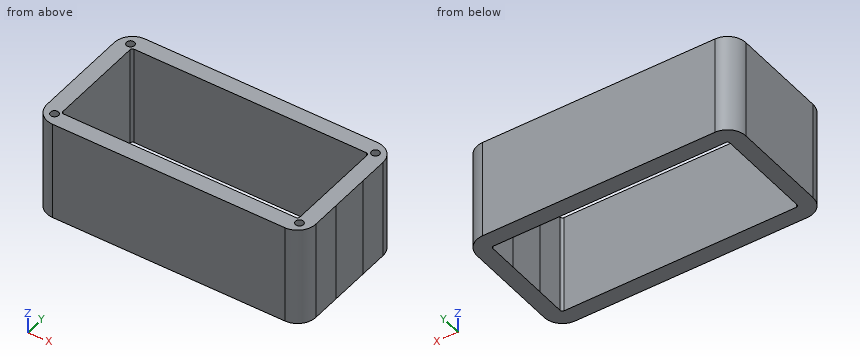
Autodesk Inventor part; units mm, degrees
ref_plane "YZ Plane" through (0, 0, 0) normal (1, 0, 0) x (0, 1, 0)
ref_plane "XZ Plane" through (0, 0, 0) normal (0, 1, 0) x (-1, 0, 0)
ref_plane "XY Plane" through (0, 0, 0) normal (0, 0, 1) x (1, 0, 0)
sketch "Sketch1" plane through (0, 0, 0) normal (0, 0, 1) x (1, 0, 0)
  line L0 (63.4168, -84.0015) -> (-66.0832, -83.9994)
  line L1 (63.4168, -84.0015) -> (81.9168, -84.0018)
  line L2 (-67.5831, -82.4994) -> (-67.5821, -20.9994)
  arc A0 (-67.5831, -82.4994) -> (-66.0832, -83.9994) centre (-66.0831, -82.4994) ccw
  arc A1 (-66.0821, -19.4994) -> (-67.5821, -20.9994) centre (-66.0821, -20.9994) ccw
  line L3 (-66.0821, -19.4994) -> (63.4179, -19.5015)
  line L4 (64.1679, -20.2516) -> (81.9179, -20.2518)
  line L5 (81.9179, -19.5018) -> (63.4179, -19.5015)
  arc A2 (83.4179, -21.0019) -> (81.9179, -19.5018) centre (81.9179, -21.0018) ccw
  line L6 (83.4176, -39.5019) -> (83.4179, -21.0019)
  line L7 (83.4176, -39.5019) -> (83.4172, -64.0019)
  line L8 (83.4169, -82.5019) -> (83.4172, -64.0019)
  arc A3 (81.9168, -84.0018) -> (83.4169, -82.5019) centre (81.9169, -82.5018) ccw
  line L9 (-77.7421, -20.9992) -> (-77.7431, -82.4992)
  arc A4 (-77.7431, -82.4992) -> (-66.0833, -94.1594) centre (-66.0831, -82.4994) ccw
  line L10 (-66.0833, -94.1594) -> (63.4167, -94.1615)
  line L11 (63.4167, -94.1615) -> (81.9167, -94.1618)
  arc A5 (81.9167, -94.1618) -> (93.5769, -82.502) centre (81.9169, -82.5018) ccw
  line L12 (93.5769, -82.502) -> (93.5772, -64.002)
  line L13 (93.5772, -64.002) -> (93.5776, -39.502)
  line L14 (93.5776, -39.502) -> (93.5779, -21.002)
  arc A6 (93.5779, -21.002) -> (81.9181, -9.3418) centre (81.9179, -21.0018) ccw
  line L15 (81.9181, -9.3418) -> (63.4181, -9.3415)
  line L16 (63.4181, -9.3415) -> (-66.0819, -9.3394)
  arc A7 (-66.0819, -9.3394) -> (-77.7421, -20.9992) centre (-66.0821, -20.9994) ccw
  point P0 (0, 0)
  dimension "d0" = 10.16
extrude "Extrusion1" add sketch "Sketch1" along normal blind 63.5
sketch "Sketch2" plane through (0, 0, 63.5) normal (0, 0, 1) x (1, 0, 0)
  circle A0 centre (-70.1221, -16.9594) radius 2.54
  circle A1 centre (85.9579, -16.9619) radius 2.54
  circle A2 centre (85.9568, -86.5419) radius 2.54
  circle A3 centre (-70.1232, -86.5394) radius 2.54
  point P0 (0, 0)
hole "Hole1" at (-70.1221, -16.9594, 63.5) at (-70.1232, -86.5394, 63.5) at (85.9579, -16.9619, 63.5) at (85.9568, -86.5419, 63.5) direction (0, 0, -1) diameter 5.08 depth 19.05
properties part number "battery hold"
The model under review builds one solid part; all positions refer to its coordinate system, in mm. Give positions to 0.01 mm unless a question says otherwise; leave off trailing zeros. Loops run counter-clockwise (first coordinate to the right, second up) from the corner with the lowest first, then second, coordinate; pieces in that order, holes last. Notation, with made-up numbers: (5, 11) -> (28, 11) arc R16 cw to (28, 32) -> close; hole circle Ø2 at (89.5, 38). An arc over 180 degrees is marked (long way). Write each question's results on one line, items separated by ' | '.
1) Take a section at D-D, the plane z = 55.5. Give the boundary of the cut face in (x, y), plus the area to 3 significant figures.
Conclusion:
outline: (-77.74, -82.5) arc R11.66 ccw to (-66.08, -94.16) -> (81.92, -94.16) arc R11.66 ccw to (93.58, -82.5) -> (93.58, -64) -> (93.58, -39.5) -> (93.58, -21) arc R11.66 ccw to (81.92, -9.34) -> (-66.08, -9.34) arc R11.66 ccw to (-77.74, -21) -> close; hole circle Ø5.08 at (-70.12, -86.54); hole circle Ø5.08 at (-70.12, -16.96); hole (-67.58, -82.5) arc R1.5 ccw to (-66.08, -84) -> (81.92, -84) arc R1.5 ccw to (83.42, -82.5) -> (83.42, -64) -> (83.42, -39.5) -> (83.42, -21) arc R1.5 ccw to (81.92, -19.5) -> (-66.08, -19.5) arc R1.5 ccw to (-67.58, -21) -> close; hole circle Ø5.08 at (85.96, -86.54); hole circle Ø5.08 at (85.96, -16.96) | area: 4,600 mm^2
2) Insertion check: pin 1 Ø4 at (x, y) = (-70, -17) entering from +Z. The pin has a flat end and moves straight along its axis. Give the tip position at first contact, or say it passes through.
Conclusion:
pin 1: stops at z = 44.45
3) For line 1 along Y through (x, z) = (-58, 22.5); line 2 along X through (y, z) = (-49, 60.5); line 3 along Y through (x, z) = (84, 61.5), list the stretches that pass through material, from the lowest coordinate up. Write a range as from..to.
Conclusion:
line 1: y = -94.16..-84, -19.5..-9.34 | line 2: x = -77.74..-67.58, 83.42..93.58 | line 3: y = -93.97..-88.16, -84.92..-18.58, -15.34..-9.53
4) Take a section at A-A, the plane z = 6.5. Give the boundary of the cut face in (x, y), plus the area to 3 significant figures.
Conclusion:
outline: (-77.74, -82.5) arc R11.66 ccw to (-66.08, -94.16) -> (81.92, -94.16) arc R11.66 ccw to (93.58, -82.5) -> (93.58, -64) -> (93.58, -39.5) -> (93.58, -21) arc R11.66 ccw to (81.92, -9.34) -> (-66.08, -9.34) arc R11.66 ccw to (-77.74, -21) -> close; hole (-67.58, -82.5) arc R1.5 ccw to (-66.08, -84) -> (81.92, -84) arc R1.5 ccw to (83.42, -82.5) -> (83.42, -64) -> (83.42, -39.5) -> (83.42, -21) arc R1.5 ccw to (81.92, -19.5) -> (-66.08, -19.5) arc R1.5 ccw to (-67.58, -21) -> close | area: 4,680 mm^2
5) Take a section at C-C, the plane x = 72. Give the boundary of the cut face in (y, z).
Conclusion:
outline: (-94.16, 0) -> (-84, 0) -> (-84, 63.5) -> (-94.16, 63.5) -> close; (-19.5, 0) -> (-9.34, 0) -> (-9.34, 63.5) -> (-19.5, 63.5) -> close
6) Take a section at B-B, the plane y = -26. Give the boundary of the cut face in (x, z), plus the area to 3 significant figures.
Conclusion:
outline: (-77.74, 0) -> (-67.58, 0) -> (-67.58, 63.5) -> (-77.74, 63.5) -> close; (83.42, 0) -> (93.58, 0) -> (93.58, 63.5) -> (83.42, 63.5) -> close | area: 1,290 mm^2
